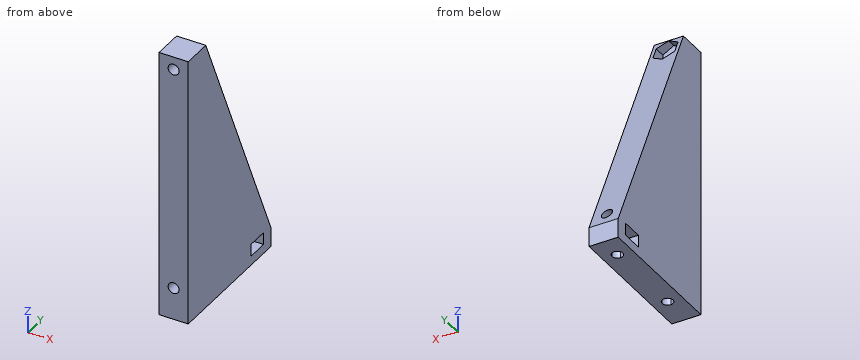
```python
from build123d import *

# Parameters (mm, degrees)
F1_DEPTH  = 13.6
F3_D      = 5.1
F5_DEPTH  = 12
F6_DEPTH  = 25
F7_DEPTH  = 15
F8_D      = 5.1
F9_W      = 5.1
F9_H      = 5.7
F10_DEPTH = 25
F4_W      = 6.8
F4_H      = 4
F11_DEPTH = 25
F12_DEPTH = 25


# Not quite as in the source:
# - a feature names something its author has since deleted; it is built from what else it names


with BuildPart() as f1:
    # F0 (on Right) → F1 (new body)
    with BuildSketch(Plane.YZ):
        Polygon((-70, 0), (0, 0), (-56, 126), (-70, 126), align=None)
        Polygon((-70, 126), (-56, 126), (-60, 135), (-70, 135), align=None)
    extrude(amount=F1_DEPTH)

    # F3 (through all)
    with Locations(Plane.XZ.offset(70)):
        with Locations((6.8, 15), (6.8, 120)):
            Hole(F3_D / 2)

    # F4 (on face) → F5 (cut)
    with BuildSketch(Plane(origin=(0, 0, 0), x_dir=(1, 0, 0), z_dir=(0, 0, -1))):
        with BuildLine():
            ThreePointArc((9.35, 55), (8.603122292, 56.803122292), (6.8, 57.55))
            Line((6.8, 57.55), (6.8, 55))
            Line((6.8, 55), (6.8, 52.45))
            ThreePointArc((6.8, 52.45), (8.603122292, 53.196877708), (9.35, 55))
        make_face()
        with BuildLine():
            ThreePointArc((9.35, 15), (8.603122292, 16.803122292), (6.8, 17.55))
            ThreePointArc((6.8, 17.55), (4.996877708, 13.196877708), (9.35, 15))
        make_face()
        with BuildLine():
            Line((6.8, 55), (6.8, 57.55))
            ThreePointArc((6.8, 57.55), (4.25, 55), (6.8, 52.45))
            Line((6.8, 52.45), (6.8, 55))
        make_face()
    extrude(amount=-F5_DEPTH, mode=Mode.SUBTRACT)

    # F2 (on face) → F6 (join)
    with BuildSketch(Plane.XZ.offset(70)):
        Polygon((11.9, 122.9444863729), (6.8, 125.8889727457), (1.7, 122.9444863729), (1.7, 117.0555136271), (6.8, 114.1110272543), (11.9, 117.0555136271), align=None)
    extrude(amount=-F6_DEPTH)

    # F7 (cut): a face of the model
    f7_faces = [f1.faces().sort_by_distance(p)[0] for p in [
        (6.8, -45, 120),
    ]]
    extrude(f7_faces, amount=-F7_DEPTH, mode=Mode.SUBTRACT)

    # F8 (through all)
    with Locations(Plane.XZ.offset(70)):
        with Locations((6.8, 120)):
            Hole(F8_D / 2)

    # F9 (on face) → F10 (cut)
    with BuildSketch(Plane(origin=(0, 0, 0), x_dir=(0, -1, 0), z_dir=(-1, 0, 0))):
        with Locations((12.45, 7.15)):
            Rectangle(F9_W, F9_H)
        with Locations((17.55, 7.15)):
            Rectangle(F9_W, F9_H)
    extrude(amount=-F10_DEPTH, mode=Mode.SUBTRACT)

    # F4 (on face) → F11 (cut)
    with BuildSketch(Plane(origin=(0, 0, 0), x_dir=(1, 0, 0), z_dir=(0, 0, -1))):
        with Locations((10.2, 2)):
            Rectangle(F4_W, F4_H)
        with Locations((3.4, 2)):
            Rectangle(F4_W, F4_H)
    extrude(amount=-F11_DEPTH, mode=Mode.SUBTRACT)

    # F0 (on Right) → F12 (cut)
    with BuildSketch(Plane.YZ):
        Polygon((-70, 126), (-56, 126), (-60, 135), (-70, 135), align=None)
    extrude(amount=F12_DEPTH, mode=Mode.SUBTRACT)


solid = f1.part
```
Read the model definition and answer for the solid it produces. Units are mm, in the model's axes. Give positions to 0.01 mm unless a question says otherwise; leave off trailing zeros. Write each loop counter-clockwise with the first axis right and the second up, starting at its lowest first coordinate (ties: lowest second). Pieces come first, ordered by that corner, then holes. Notation, with made-up numbers: M 10,-7.75 L 65,-7.75 A19 cw 65,10.25 Z; hole C 27.5,88 d2. An arc over 180 degrees is marked long. Put each result on its own line as item: value. Start each with the question number.
1. The part is cut by section C-C, the plane x = 8. Give the number of separate pieces and of enclosed holes in the cut face, and give its area (3 significant figures).
2. The part is cut by section A-A, the plane y = -26. Give the vertices of the cut face in (x, z).
3. The part is cut by section B-B, the plane z = 120. Give the vertices of the cut face in (x, y), and give its area (3 significant figures).
4. Consider line 1 along Y through (x, z) = (6.8, 1.55); line 2 along X through (y, z) = (-15, 1); line 3 along Z through (x, y) = (6.8, -63.25). Determine where each line is inside the solid, lowest interval first.
5. The part is cut by section D-D, the plane z = 15. Give the vertices of the cut face in (x, y).
6. Each of these flat-tipped pins is pushed along its axis until it touches: pin 1 Ø4.5 at (x, y) = (6.8, -15) entering from +Z; pin 2 Ø5 at (x, z) = (1.5, 39.5) entering from +Y; pin 3 Ø2.5 at (x, y) = (6.5, -15.5) entering from -Z; pin 4 Ø4.5 at (x, z) = (6.8, 15) entering from +Y. Where does it stop, or does it pass through?
Final values:
1. separate pieces: 3
1. enclosed holes: 0
1. area: 4,730 mm²
2. outline: M 0,0 L 13.6,0 L 13.6,58.5 L 0,58.5 Z; hole C 6.8,15 d5.1
3. outline: M 0,-70 L 4.25,-70 L 4.25,-60 L 1.7,-60 L 1.7,-53.33 L 0,-53.33 Z; M 9.35,-70 L 13.6,-70 L 13.6,-53.33 L 11.9,-53.33 L 11.9,-60 L 9.35,-60 Z
3. area: 108 mm²
4. line 1: y = -70 to -57.55, -52.45 to -17.55, -12.45 to -4
4. line 2: x = 0 to 4.25, 9.35 to 13.6
4. line 3: z = 0 to 12.45, 17.55 to 117.45, 122.55 to 126
5. outline: M 0,-70 L 4.25,-70 L 4.25,-6.67 L 0,-6.67 Z; M 9.35,-70 L 13.6,-70 L 13.6,-6.67 L 9.35,-6.67 Z
6. pin 1: stops at z = 38.81
6. pin 2: stops at y = -16.44
6. pin 3: stops at z = 12
6. pin 4: passes through
